The figure shows three views and two pictorial views of one solid part (mm, origin at its lowest corner). Answer the questions. A direction names the side the tool comes from. Coordinates: 2 decimals unless noted, no trailing zeros. Order: outer loops, then holes, each group sorted by start corner. A loop starts at its lowest first (then second) coordinate and runs counter-clockwise, first axis right, second up.
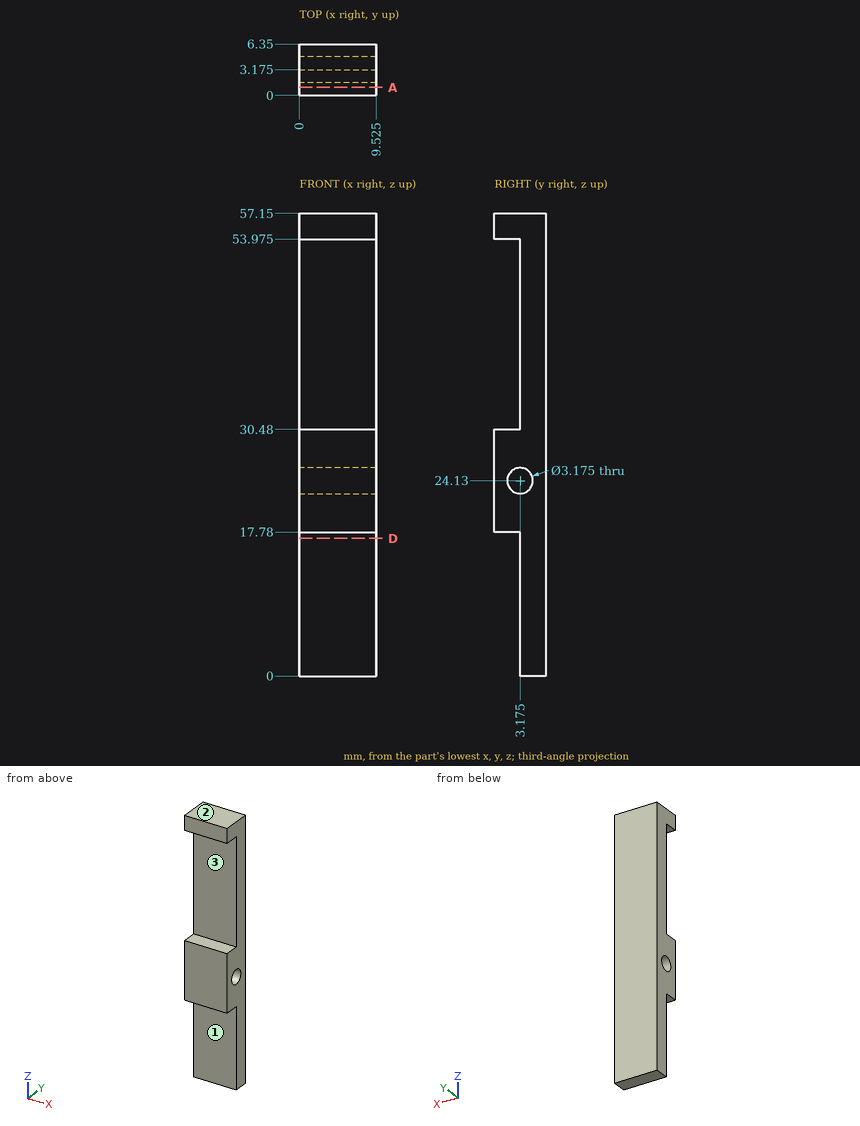
Q1. Straight lines are drawn through the part: L1, parallel to Z at x = 8.25, y = 1.5 (3 decimals); L2, parallel to Y at x = 3.25, z = 24.13; L3, parallel to Z at x = 8.25, y = 3.25. For each, find the intervals that lie inside material, in ascending order.
Q2. The part is cut by section A-A, the plane y = 1. Determine the outline of the cut face in (x, z) (3 decimals), then the cut area to 3 significant figures.
Q3. The part is cut by section D-D, the plane z = 17. Determine the outline of the cut face in (x, y) (3 decimals).
Q4. Each of these flat-tipped pins is pushed along its axis until it touches: P1, Ø2.5, axis at x = 6, y = 1.5, coming from the -Z side; P2, Ø4, axis at x = 7, z = 16.5, coming from the -Y side; P3, Ø5, axis at x = 5, z = 42, coming from the -Y side (3 decimals). Where does it stop, or does it pass through?
Q5. Which of the six approach directions +Z, -Z, +X, -X, +Y, -Y give full straight-line access (tool end or side, diameter ignored) to the marked faces 1, 2 and 3?
Computed values:
1. L1: z = 17.78 to 30.48, 53.975 to 57.15
1. L2: y = 0 to 1.59, 4.76 to 6.35
1. L3: z = 0 to 22.54, 25.72 to 57.15
2. outline: (0, 17.78) - (9.525, 17.78) - (9.525, 30.48) - (0, 30.48) - close; (0, 53.975) - (9.525, 53.975) - (9.525, 57.15) - (0, 57.15) - close
2. area: 151 mm2
3. outline: (0, 3.175) - (9.525, 3.175) - (9.525, 6.35) - (0, 6.35) - close
4. P1: stops at z = 17.78
4. P2: stops at y = 0
4. P3: stops at y = 3.175
5. face 1: -Z, +X, -X, -Y
5. face 2: +Z, +X, -X, +Y, -Y
5. face 3: +X, -X, -Y
